```python
from build123d import *

# Parameters (mm, degrees)
SKETCH1_R               = 37.592
BOSS_EXTRUDE1_DEPTH     = 50.8
SKETCH4_R               = 37.592
BOSS_EXTRUDE2_DEPTH     = 50.8
SKETCH5_R               = 6.25475
SKETCH5_R_2             = 4.22275
BOSS_EXTRUDE3_DEPTH     = 101.6
CUT_EXTRUDE1_DEPTH      = 60.198
CUT_EXTRUDE1_DEPTH_BACK = 64.516
SKETCH6_W               = 13.208
SKETCH6_H               = 76.2


with BuildPart() as part:
    # Sketch1 → Boss-Extrude1 (new body)
    with BuildSketch(Plane(origin=(0, 0, 0), x_dir=(1, 0, 0), z_dir=(0, 1, 0))):
        with Locations(Location((0, 0, 0), (0, 0, 270))):
            Circle(SKETCH1_R)
        with BuildLine():
            Line((-35.143970714, 1.272475327), (-35.143970714, -0.505524673))
            Line((-35.143970714, -0.505524673), (-31.004836055, -0.505524673))
            Line((-31.004836055, -0.505524673), (-31.004836055, -3.045524673))
            Line((-31.004836055, -3.045524673), (-33.544836055, -3.045524673))
            ThreePointArc((-33.544836055, -3.045524673), (0, -33.682803423), (33.544836055, -3.045524673))
            Line((33.544836055, -3.045524673), (31.004836055, -3.045524673))
            Line((31.004836055, -3.045524673), (31.004836055, -0.505524673))
            Line((31.004836055, -0.505524673), (35.143970714, -0.505524673))
            Line((35.143970714, -0.505524673), (35.143970714, 1.272475327))
            Line((35.143970714, 1.272475327), (30.926345458, 1.272475327))
            Line((30.926345458, 1.272475327), (30.926345458, 3.812475327))
            Line((30.926345458, 3.812475327), (33.466345458, 3.812475327))
            ThreePointArc((33.466345458, 3.812475327), (0, 33.682803423), (-33.466345458, 3.812475327))
            Line((-33.466345458, 3.812475327), (-30.926345458, 3.812475327))
            Line((-30.926345458, 3.812475327), (-30.926345458, 1.272475327))
            Line((-30.926345458, 1.272475327), (-35.143970714, 1.272475327))
        make_face(mode=Mode.SUBTRACT)
    extrude(amount=BOSS_EXTRUDE1_DEPTH)

    # Sketch4 → Boss-Extrude2 (add)
    with BuildSketch(Plane(origin=(0, 50.8, 0), x_dir=(1, 0, 0), z_dir=(0, 1, 0))):
        with Locations(Location((0, 0, 0), (0, 0, 270))):
            Circle(SKETCH4_R)
        with BuildLine():
            Line((33.466345458, 3.812475327), (-33.466345458, 3.812475327))
            ThreePointArc((-33.466345458, 3.812475327), (0, 33.682803423), (33.466345458, 3.812475327))
        make_face(mode=Mode.SUBTRACT)
        with BuildLine():
            Line((-30.926345458, 1.272475327), (30.926345458, 1.272475327))
            Line((30.926345458, 1.272475327), (30.965590757, 0.383475327))
            Line((30.965590757, 0.383475327), (33.680620439, 0.383475327))
            ThreePointArc((33.680620439, 0.383475327), (0, -33.682803423), (-33.680620439, 0.383475327))
            Line((-33.680620439, 0.383475327), (-30.965590757, 0.383475327))
            Line((-30.965590757, 0.383475327), (-30.926345458, 1.272475327))
        make_face(mode=Mode.SUBTRACT)
    extrude(amount=BOSS_EXTRUDE2_DEPTH)

    # Sketch5 → Boss-Extrude3 (add)
    # profile 1 of 2: a face of its own
    with BuildSketch(Plane.XZ):
        with Locations((0, -29.670562634)):
            Circle(SKETCH5_R)
        with Locations((0, -29.670562634)):
            Circle(SKETCH5_R_2, mode=Mode.SUBTRACT)
    # profile 2 of 2: a face of its own
    with BuildSketch(Plane.XZ):
        with Locations((0, 29.670562634)):
            Circle(SKETCH5_R)
        with Locations((0, 29.670562634)):
            Circle(SKETCH5_R_2, mode=Mode.SUBTRACT)
    extrude(amount=-BOSS_EXTRUDE3_DEPTH)

    # Sketch6 → Cut-Extrude1 (cut, two sides: drawn at the far end of the back side and taken through both)
    with BuildSketch(Plane(origin=(0, 0, 0), x_dir=(0, 0, -1), z_dir=(1, 0, 0)).offset(-CUT_EXTRUDE1_DEPTH_BACK)):
        with Locations((10.416475327, 58.42)):
            Rectangle(SKETCH6_W, SKETCH6_H)
    extrude(amount=CUT_EXTRUDE1_DEPTH + CUT_EXTRUDE1_DEPTH_BACK, mode=Mode.SUBTRACT)


solid = part.part
```
Input: part model. Units: mm. Frame: model coordinates. A direction names the side the tool comes from. Round coordinates to 2 decimals unless told otherwise and drop trailing zeros. Loops run counter-clockwise (first coordinate to the right, second up) from the corner with the lowest first, then second, coordinate; pieces in that order, holes last. Notation, with made-up numbers: (74.25, 62.25) - (133.25, 62.25) arc R22 ccw to (133.25, 91.25) - close; hole circle Ø1 at (-5.5, 16.25). An arc over 180 degrees is marked (long way). One line per item, written item: value. Start each with the question number.
(1) Section C-C, the plane x = 0. Return loops of the section in (y, z), plus the area to 3 significant figures.
(2) Section D-D, the plane y = 6.5. Return loops of the section in (x, z), plus the area to 3 significant figures.
(3) Draft query along X for faces 4 (the flat face through (32, 25, 3.046)), 5 (the cylindrical face through (11.292, 50.089, 35.856)), 6 (the flat face through (-31, 58, -17.02)). Return one class per face: +X half, -X half, draft (parallel to the pull), parting line (faces both ways), or undercut.
(4) Section A-A, the plane y = 68. Return loops of the section in (x, z), plus the area to 3 significant figures.
(5) Ray query, line 1 (X direction, y = 80.5, z = 29.5); line 2 (X direction, y = 17, z = -30); line 3 (Z direction, x = -6.5, y = 52). Return the intervals inside material, ascending. Write a range as [from, to].
(6) Contact query for flat-ended pins moving along their axis: P1, Ø3, axis at y = 17.5, z = -3, coming from the -X side; P2, Ø2, axis at y = 55.5, z = 24.5, coming from the +X side; P3, Ø4.5, axis at x = 33.5, y = 19.5, coming from the -Z side. Output: stop coordinate, or through.
(7) Section B-B, the plane y = 37. Return loops of the section in (x, z), plus the area to 3 significant figures.
(8) Access query for faces 1 (the flat face through (32, 76, -0.383)), 2 (the flat face through (-33, 25, -1.272)), 3 (the flat face through (-34, 20.32, -10)). Directions: +Z, -Z, +X, -X, +Y, -Y. A direction counts if a zero-diameter tool reaches every point of the face in a straight line with its end or side. Return the directions, or none.
Results below:
1. outline: (0, -37.59) - (101.6, -37.59) - (101.6, -33.68) - (0, -33.68) - close; (0, -25.45) - (101.6, -25.45) - (101.6, -23.42) - (0, -23.42) - close; (0, 23.42) - (101.6, 23.42) - (101.6, 25.45) - (0, 25.45) - close; (0, 33.68) - (101.6, 33.68) - (101.6, 37.59) - (0, 37.59) - close; (50.8, -3.81) - (101.6, -3.81) - (101.6, -1.27) - (50.8, -1.27) - close
1. area: 1,340 mm^2
2. outline: circle Ø75.18 at (0, 0); hole (-35.14, -1.27) - (-30.93, -1.27) - (-30.93, -3.81) - (-33.47, -3.81) arc R33.68 ccw to (-5.1, -33.29) arc R6.25 cw (long way) to (5.1, -33.29) arc R33.68 ccw to (33.47, -3.81) - (30.93, -3.81) - (30.93, -1.27) - (35.14, -1.27) - (35.14, 0.51) - (31, 0.51) - (31, 3.05) - (33.54, 3.05) arc R33.68 ccw to (5.1, 33.29) arc R6.25 cw (long way) to (-5.1, 33.29) arc R33.68 ccw to (-33.54, 3.05) - (-31, 3.05) - (-31, 0.51) - (-35.14, 0.51) - close; hole (-1.4, -33.65) arc R33.68 ccw to (1.4, -33.65) arc R4.22 ccw (long way) to start; hole (-1.4, 33.65) arc R4.22 ccw (long way) to (1.4, 33.65) arc R33.68 ccw to start
2. area: 999 mm^2
3. face 4: undercut
3. face 5: parting line
3. face 6: draft
4. outline: (-37.4, -3.81) - (37.4, -3.81) arc R37.59 ccw (long way) to start; (-33.52, -17.02) arc R37.59 ccw to (33.52, -17.02) - (29.07, -17.02) arc R33.68 cw to (5.1, -33.29) arc R6.25 ccw (long way) to (-5.1, -33.29) arc R33.68 cw to (-29.07, -17.02) - close; hole (-33.68, -0.38) - (-30.97, -0.38) - (-30.93, -1.27) - (30.93, -1.27) - (30.97, -0.38) - (33.68, -0.38) arc R33.68 ccw to (5.1, 33.29) arc R6.25 cw (long way) to (-5.1, 33.29) arc R33.68 ccw to start; hole (-1.4, -33.65) arc R33.68 ccw to (1.4, -33.65) arc R4.22 ccw (long way) to start; hole (-1.4, 33.65) arc R4.22 ccw (long way) to (1.4, 33.65) arc R33.68 ccw to start
4. area: 1,040 mm^2
5. line 1: [-23.3, -16.26], [-6.25, -4.22], [4.22, 6.25], [16.26, 23.3]
5. line 2: [-22.65, -15.31], [-6.25, -4.21], [4.21, 6.25], [15.31, 22.65]
5. line 3: [-37.03, -33.05], [-3.81, -1.27], [33.05, 37.03]
6. P1: x = -37.56
6. P2: x = 29.34
6. P3: z = -20.89
7. outline: (-37.4, -3.81) - (-30.93, -3.81) - (-30.93, -1.27) - (-35.14, -1.27) - (-35.14, 0.51) - (-31, 0.51) - (-31, 3.05) - (-33.54, 3.05) arc R33.68 cw to (-5.1, 33.29) arc R6.25 ccw (long way) to (5.1, 33.29) arc R33.68 cw to (33.54, 3.05) - (31, 3.05) - (31, 0.51) - (35.14, 0.51) - (35.14, -1.27) - (30.93, -1.27) - (30.93, -3.81) - (37.4, -3.81) arc R37.59 ccw (long way) to start; (-33.52, -17.02) arc R37.59 ccw to (33.52, -17.02) - (29.07, -17.02) arc R33.68 cw to (5.1, -33.29) arc R6.25 ccw (long way) to (-5.1, -33.29) arc R33.68 cw to (-29.07, -17.02) - close; hole (-1.4, -33.65) arc R33.68 ccw to (1.4, -33.65) arc R4.22 ccw (long way) to start; hole (-1.4, 33.65) arc R4.22 ccw (long way) to (1.4, 33.65) arc R33.68 ccw to start
7. area: 890 mm^2
8. face 1: +Y, -Y
8. face 2: -Y
8. face 3: +X, -X
